Input: part model. Units: mm. Frame: model coordinates. Face numbers are marked on the shaded views. Give positions to 0.01 mm unless a question says otherwise; leave off trailing zeros. Order: outer loops, then holes, each group sorted by start corner. A loop starts at its lowest first (then second) coordinate and runs counter-clockwise, first axis right, second up. Notation, with made-up numbers: (-23.5, 44.25) - (-11.5, 44.25) arc R8 ccw to (-11.5, 49.25) - close; hole circle Ø6 at (56, 83.5). An arc over 180 degrees is marked (long way). Use a Markdown table: item, result.
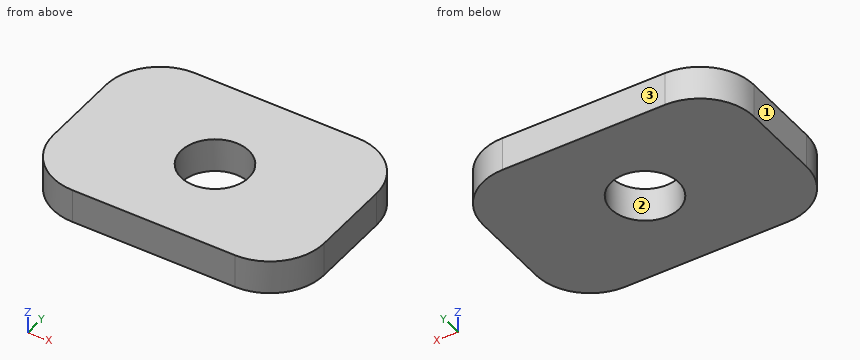
from build123d import *

# Parameters (mm, degrees)
SKETCH1_W           = 25.4
SKETCH1_H           = 17.78
BOSS_EXTRUDE1_DEPTH = 3.175
HOLE1_D             = 6.35
FILLET1_R           = 5.08


with BuildPart() as part:
    # Sketch1 → Boss-Extrude1 (new body)
    with BuildSketch(Plane.XY):
        with Locations((12.7, -8.89)):
            Rectangle(SKETCH1_W, SKETCH1_H)
    extrude(amount=BOSS_EXTRUDE1_DEPTH)

    # Hole1 (through all)
    with Locations(Plane.XY.offset(3.175)):
        with Locations((12.7, -8.89)):
            Hole(HOLE1_D / 2)

    # Fillet1
    fillet1_edges = [part.edges().sort_by_distance(p)[0] for p in [
        (0, 0, 1.5875),
        (25.4, 0, 1.5875),
        (25.4, -17.78, 1.5875),
        (0, -17.78, 1.5875),
    ]]
    fillet(fillet1_edges, radius=FILLET1_R)


solid = part.part
1. Section query A-A (y = -8.89). Return loops of the section in (x, z) (3 decimals), then the cut area to 3 significant figures.
Response:
| item | result |
|---|---|
| outline | (0, 0) - (9.525, 0) - (9.525, 3.175) - (0, 3.175) - close; (15.875, 0) - (25.4, 0) - (25.4, 3.175) - (15.875, 3.175) - close |
| area | 60.5 mm^2 |
2. Section query B-B (x = 12.7). Return loops of the section in (y, z) (3 decimals).
Response:
| item | result |
|---|---|
| outline | (-17.78, 0) - (-12.065, 0) - (-12.065, 3.175) - (-17.78, 3.175) - close; (-5.715, 0) - (0, 0) - (0, 3.175) - (-5.715, 3.175) - close |
3. Mould query, pull axis Y, two halves, no side actions, for the marked faces 1, 2 and 3. Classes: pulls with the +Y half, pulls with the -Y half, needs draft (parallel to the pull), parting line crosses it, or undercut.
Response:
| item | result |
|---|---|
| face 1 | needs draft |
| face 2 | undercut |
| face 3 | pulls with the +Y half |
4. Section query D-D (x = 23.25). Return loops of the section in (y, z) (3 decimals).
Response:
| item | result |
|---|---|
| outline | (-16.85, 0) - (-0.93, 0) - (-0.93, 3.175) - (-16.85, 3.175) - close |
5. Material intervals for line 1 along Y through (x, z) = (12.7, 1) (3 decimals); line 2 along X through (y, z) = (-9, 0.65); line 3 along X through (y, z) = (-8, 1.1), sorted ascending.
Response:
| item | result |
|---|---|
| line 1 | y = -17.78 to -12.065, -5.715 to 0 |
| line 2 | x = 0 to 9.53, 15.87 to 25.4 |
| line 3 | x = 0 to 9.65, 15.75 to 25.4 |
6. Section query C-C (z = 2.35). Return loops of the section in (x, y) (3 decimals), then the cut area to 3 significant figures.
Response:
| item | result |
|---|---|
| outline | (0, -12.7) arc R5.08 ccw to (5.08, -17.78) - (20.32, -17.78) arc R5.08 ccw to (25.4, -12.7) - (25.4, -5.08) arc R5.08 ccw to (20.32, 0) - (5.08, 0) arc R5.08 ccw to (0, -5.08) - close; hole circle Ø6.35 at (12.7, -8.89) |
| area | 398 mm^2 |
